Autodesk Inventor part; units mm, degrees
ref_plane "YZ Plane" through (0, 0, 0) normal (1, 0, 0) x (0, 1, 0)
ref_plane "XZ Plane" through (0, 0, 0) normal (0, 1, 0) x (-1, 0, 0)
ref_plane "XY Plane" through (0, 0, 0) normal (0, 0, 1) x (1, 0, 0)
sketch "Szkic1" plane through (0, 0, 0) normal (0, 1, 0) x (-1, 0, 0)
  line L0 (0, 0) -> (90, 0)
  line L1 (90, 0) -> (90, -60)
  line L2 (90, -60) -> (0, -60)
  line L3 (0, -60) -> (0, 0)
  dimension "d0" = 90
  dimension "d1" = 60
extrude "Wyciągnięcie proste1" add sketch "Szkic1" along normal blind 2
sketch "Szkic10" plane through (0, 2, 0) normal (0, 1, 0) x (1, 0, 0)
  circle A0 centre (-83, 54.5) radius 3
  circle A1 centre (-25, 54.5) radius 3
  circle A2 centre (-25, 5.5) radius 3
  circle A3 centre (-83, 5.5) radius 3
  point P0 (0, 0)
  dimension "d21" = 6
  dimension "d22" = 6
  dimension "d23" = 6
  dimension "d24" = 6
extrude "Wyciągnięcie proste4" add sketch "Szkic10" along normal blind 6
sketch "Szkic11" plane through (-83, 8, -54.5) normal (0, 1, 0) x (1, 0, 0)
  circle A0 centre (0, 0) radius 3
  point P0 (83, -54.5)
hole "Otwór1" at (-83, 8, -54.5) direction (0, -1, 0) diameter 2.1129 depth 4 tip angle 118 counterbore diameter 2.7 counterbore depth 0
sketch "Szkic12" plane through (-83, 8, -5.5) normal (0, 1, 0) x (1, 0, 0)
  circle A0 centre (0, 0) radius 3
  point P0 (83, -5.5)
hole "Otwór2" at (-83, 8, -5.5) direction (0, -1, 0) diameter 2.1129 depth 4 tip angle 118 counterbore diameter 2.7 counterbore depth 0
sketch "Szkic13" plane through (-25, 8, -54.5) normal (0, 1, 0) x (1, 0, 0)
  point P0 (25, -54.5)
  point P1 (0, 0)
  point P2 (0, 0)
hole "Otwór3" at (-25, 8, -54.5) direction (0, -1, 0) diameter 2.1129 depth 4 tip angle 118 counterbore diameter 2.7 counterbore depth 0
sketch "Szkic14" plane through (-25, 8, -5.5) normal (0, 1, 0) x (1, 0, 0)
  point P0 (25, -5.5)
  point P1 (0, 0)
  point P2 (0, 0)
hole "Otwór4" at (-25, 8, -5.5) direction (0, -1, 0) diameter 2.1129 depth 4 tip angle 118 counterbore diameter 2.7 counterbore depth 0
sketch "Szkic15" plane through (-90, 0, -60) normal (-1, 0, 0) x (0, 0, 1)
  line L0 (0, 0) -> (60, 0)
  line L1 (60, 0) -> (60, 2)
  line L2 (60, 2) -> (0, 2)
  line L3 (0, 2) -> (0, 0)
extrude "Wyciągnięcie proste5" add sketch "Szkic15" along normal blind 5
sketch "Szkic16" plane through (0, 2, 0) normal (0, 1, 0) x (1, 0, 0)
  line L0 (0, 60) -> (-95, 60)
  line L1 (-95, 60) -> (-95, 0)
  line L2 (-94, 60) -> (-95, 60)
  line L3 (-95, 60) -> (-95, 0)
  line L4 (-95, 0) -> (-94, 0)
  line L5 (-94, 0) -> (-94, 60)
  line L6 (-95, 1) -> (0, 1)
  line L7 (0, 1) -> (0, 0)
  line L8 (0, 0) -> (-95, 0)
  line L9 (-95, 0) -> (-95, 1)
  line L10 (-1, 0) -> (0, 0)
  line L11 (0, 0) -> (0, 60)
  line L12 (0, 60) -> (-1, 60)
  line L13 (-1, 60) -> (-1, 0)
  line L14 (-1, 59) -> (-95, 59)
  line L15 (-95, 59) -> (-95, 60)
  line L16 (-95, 60) -> (-1, 60)
  line L17 (-1, 60) -> (-1, 59)
  point P0 (-94, 59)
  point P1 (-1, 1)
  point P2 (-94, 1)
extrude "Wyciągnięcie proste6" add sketch "Szkic16" along normal blind 8 contours L11 L6 L13 L0 | L13 L14 L5 L0 | L7 L8 L13 L6 | L5 L14 L1 L0 | L13 L8 L5 L6 | L5 L6 L1 L14 | L5 L4 L1 L6
sketch "Szkic21" plane through (0, 2, 0) normal (0, 1, 0) x (1, 0, 0)
  line L0 (-1, 59) -> (-1, 1)
  line L1 (-94, 1) -> (-1, 1)
  line L2 (-1, 5) -> (-5, 5)
  line L3 (-5, 5) -> (-5, 1)
  line L4 (-5, 1) -> (-1, 1)
  line L5 (-1, 1) -> (-1, 5)
  point P0 (0, 0)
  dimension "d61" = 4
extrude "Wyciągnięcie proste8" add sketch "Szkic21" along normal blind 8
sketch "Szkic22" plane through (0, 2, 0) normal (0, 1, 0) x (1, 0, 0)
  line L0 (-1, 59) -> (-1, 5)
  line L1 (-1, 55) -> (-5, 55)
  line L2 (-5, 55) -> (-5, 59)
  line L3 (-5, 59) -> (-1, 59)
  line L4 (-1, 59) -> (-1, 55)
  line L5 (-94, 1) -> (-94, 59)
  line L6 (-1, 59) -> (-94, 59)
  line L7 (-94, 55) -> (-90, 55)
  line L8 (-90, 55) -> (-90, 59)
  line L9 (-90, 59) -> (-94, 59)
  line L10 (-94, 59) -> (-94, 55)
  line L11 (-94, 1) -> (-5, 1)
  line L12 (-94, 5) -> (-90, 5)
  line L13 (-90, 5) -> (-90, 1)
  line L14 (-90, 1) -> (-94, 1)
  line L15 (-94, 1) -> (-94, 5)
  point P0 (0, 0)
  dimension "d64" = 4
  dimension "d65" = 4
extrude "Wyciągnięcie proste9" add sketch "Szkic22" along normal blind 8
fillet "Zaokrąglenie1" radius 2 4 edges at (-90, 6, -55) (-5, 6, -55) (-90, 6, -5) (-5, 6, -5)
sketch "Szkic23" plane through (0, 10, 0) normal (0, 1, 0) x (1, 0, 0)
  point P0 (0, 0)
  point P1 (-2.5, 2.5)
  point P2 (-92.5, 2.5)
  point P3 (-92.5, 57.5)
  point P4 (-2.5, 57.5)
hole "Otwór5" at (-2.5, 10, -2.5) at (-92.5, 10, -2.5) at (-92.5, 10, -57.5) at (-2.5, 10, -57.5) direction (0, -1, 0) diameter 2.1129 depth 4 tip angle 118 counterbore diameter 2.7 counterbore depth 0
equation "\"d25\" = d22"
properties part number "dol"
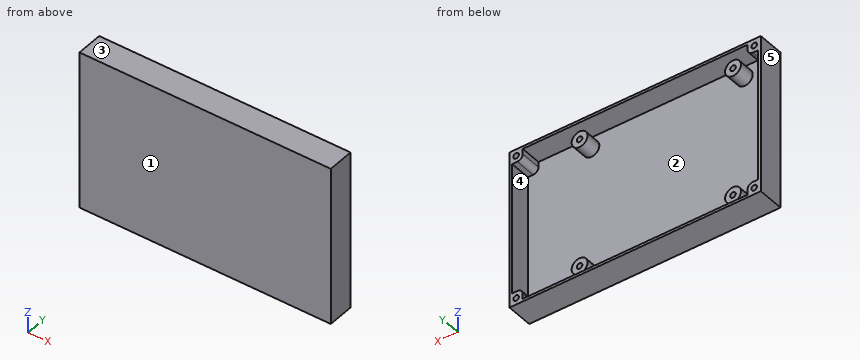
Work out the finished part from the listing and answer in its coordinate system (mm). Face numbers are marked on the shaded views. A direction names the side the tool comes from. Give positions to 0.01 mm unless a question says otherwise; leave off trailing zeros. Loops run counter-clockwise (first coordinate to the right, second up) from the corner with the lowest first, then second, coordinate; pieces in that order, holes last. Notation, with made-up numbers: (46.5, 4.5) -> (63.5, 4.5) arc R29 ccw to (63.5, 36.5) -> close; hole circle Ø4 at (-6.5, 77.5). An arc over 180 degrees is marked (long way). One line per question, with ' | ' between items. Start each with the question number.
1) Straight lines are drawn through the part: L1, parallel to Z at x = -2.5, y = 8.55; L2, parallel to Z at x = -25, y = 5.55; L3, parallel to X at y = 4.75, z = -5.5. For each, find the intervals that lie inside material, in ascending order.
2) Each of these flat-tipped pins is pushed along its axis until it touches: pin 1 (2 mm diameter, centred on x = -20, z = -31.5, fed in from +Y); pin 2 (1.3 mm diameter, centred on x = -83, z = -54.5, fed in from +Y); pin 3 (5 mm diameter, centred on x = -84, z = -6, fed in from +Y). Where does it stop, or does it pass through?
3) Section B-B, the plane x = -58 is taken. Determine the outline of the cut face in (y, z), then the cut area to 3 significant figures.
4) Section A-A, the plane z = -20.5 is taken. Determine the outline of the cut face in (x, y).
5) Determine the mould class of the marked faces 1, 2 and 3 for opening direction Z: +Z half, -Z half, draft (parallel to the pull), parting line (faces both ways), or undercut.
6) For the marked faces 4 and 5, determine the directions among +Z, -Z, +X, -X, +Y, -Y from which every point of the face is accessible in a straight line to the end or side of a thin tool.
Resolved:
1) L1: -60 to -58.56, -56.44 to -55, -5 to -3.56, -1.44 to 0 | L2: -60 to -59, -57.5 to -55.56, -53.44 to -51.5, -8.5 to -6.56, -4.44 to -2.5, -1 to 0 | L3: -95 to -94, -86 to -84.06, -81.94 to -80, -28 to -26.06, -23.94 to -22, -1 to 0
2) pin 1: y = 2 | pin 2: y = 3.76 | pin 3: y = 8
3) outline: (0, -60) -> (10, -60) -> (10, -59) -> (2, -59) -> (2, -1) -> (10, -1) -> (10, 0) -> (0, 0) -> close | area: 136 mm2
4) outline: (-95, 0) -> (0, 0) -> (0, 10) -> (-1, 10) -> (-1, 2) -> (-94, 2) -> (-94, 10) -> (-95, 10) -> close
5) face 1: draft | face 2: undercut | face 3: +Z half
6) face 4: +Y | face 5: +Z, -Z, -X, +Y, -Y
